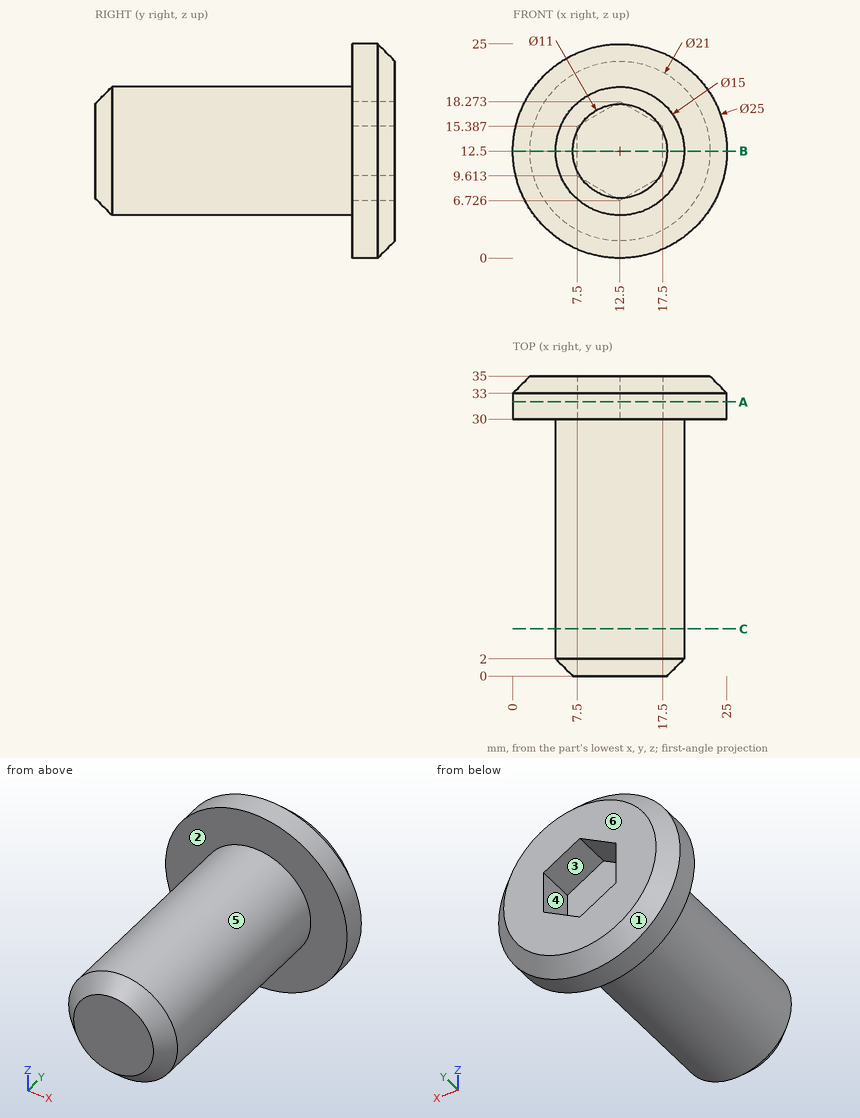
Geometry check sheet. Reference: drawing and pictorial views, mm from the part's lowest x, y, z. A direction names the side the tool comes from. Coordinates: 2 decimals unless noted, no trailing zeros. Loops run counter-clockwise (first coordinate to the right, second up) from the corner with the lowest first, then second, coordinate; pieces in that order, holes last. Notation, with made-up numbers: M 1.5,-31.5 L 35.5,-31.5 A19 cw 35.5,-15.5 Z; hole C 62,18 d5. An arc over 180 degrees is marked long. One line per item, written item: value.
1. Gauge pin test, flat ends, axial feed: P1, Ø3, axis at x = 8.5, y = 31, coming from the -Z side; P2, Ø3, axis at y = 17.5, z = 5.5, coming from the -X side; P3, Ø5, axis at y = 29, z = 8.5, coming from the -X side. Record the tip position at first contact, or that the pin passes through.
Answers follow:
P1: z = 0.25
P2: x = 7.4
P3: x = 0.12
2. Set-up check for the marked faces 4, 5 and 6: record each of +Z, -Z, +X, -X, +Y, -Y from which the full face is reachable in a straight line by a thin tool's end or side.
Answers follow:
face 4: +Y
face 5: -Y
face 6: +Z, -Z, +X, -X, +Y
3. Mould release check, pull along Z, two halves, no side actions. Record for the marked faces 1, 2 and 3: pulls with the +Z half, pulls with the -Z half, needs draft (parallel to the pull), parting line crosses it, or undercut.
Answers follow:
face 1: parting line crosses it
face 2: needs draft
face 3: undercut
4. Material ranges on line 1 along Y through (x, z) = (13.75, 21.25); line 2 along Z through (x, y) = (12.75, 23) (1 decimal); line 3 along Z through (x, y) = (8.5, 32) (1 decimal), recorded low to high. Write a range as from..to.
Answers follow:
line 1: 30..35
line 2: 5..20
line 3: 0.7..9, 16..24.3
5. Section check B-B on z = 12.5. Record the cut outline in (x, y).
Answers follow:
outline: M 0,30 L 5,30 L 5,2 L 7,0 L 18,0 L 20,2 L 20,30 L 25,30 L 25,33 L 23,35 L 17.5,35 L 17.5,30 L 7.5,30 L 7.5,35 L 2,35 L 0,33 Z
6. Section check C-C on y = 5.5. Record the cut outline in (x, z), plus the area to 3 significant figures.
Answers follow:
outline: C 12.5,12.5 d15
area: 177 mm^2
7. Section check A-A on y = 32. Record the cut outline in (x, z), plus the area to 3 significant figures.
Answers follow:
outline: C 12.5,12.5 d25; hole M 7.5,9.61 L 12.5,6.73 L 17.5,9.61 L 17.5,15.39 L 12.5,18.27 L 7.5,15.39 Z
area: 404 mm^2
